The model under review builds one solid part; all positions refer to its coordinate system, in mm. Coordinates: 2 decimals unless noted, no trailing zeros. Loops run counter-clockwise (first coordinate to the right, second up) from the corner with the lowest first, then second, coordinate; pieces in that order, holes last. Notation, with made-up numbers: M 57.5,-14 L 89.5,-14 A27 cw 89.5,8 Z; hole C 4.25,66 d2. An arc over 180 degrees is marked long. Return JSON: item names as keys, results as strings.
```python
from build123d import *

# Parameters (mm, degrees)
F2_DEPTH = 11
F4_DEPTH = 7.1505523714


with BuildPart() as f2:
    # F1 (on Front) → F2 (new body)
    with BuildSketch(Plane.XZ):
        with BuildLine():
            Line((14.506585896, 14), (14.506585896, 20.0424585491))
            Line((14.506585896, 20.0424585491), (-19.4195080549, 20.0424585491))
            Line((-19.4195080549, 20.0424585491), (-19.4195080549, -20.0424585491))
            Line((-19.4195080549, -20.0424585491), (14.506585896, -20.0424585491))
            Line((14.506585896, -20.0424585491), (14.506585896, -14))
            Line((14.506585896, -14), (0, -14))
            ThreePointArc((0, -14), (-14, 0), (0, 14))
            Line((0, 14), (14.506585896, 14))
        make_face()
    extrude(amount=F2_DEPTH)

    # F3 (on face) → F4 (cut, through all)
    with BuildSketch(Plane(origin=(0, 0, -20.0424585491), x_dir=(1, 0, 0), z_dir=(0, 0, -1))):
        with BuildLine():
            Line((-2.4564610794, 8.5), (-2.4564610794, 2.5))
            ThreePointArc((-2.4564610794, 2.5), (-0.3351407359, 3.3786796564), (0.5435389206, 5.5))
            ThreePointArc((0.5435389206, 5.5), (-0.3351407359, 7.6213203436), (-2.4564610794, 8.5))
        make_face()
        with BuildLine():
            ThreePointArc((-2.4564610794, 8.5), (-5.4564610794, 5.5), (-2.4564610794, 2.5))
            Line((-2.4564610794, 2.5), (-2.4564610794, 8.5))
        make_face()
    extrude(amount=-F4_DEPTH, mode=Mode.SUBTRACT)


solid = f2.part
```
1. Add section C-C on y = -5. Give the boundary of the cut face in (x, z), plus the area to 3 significant figures.
Check values:
{"outline": "M -19.42,-20.04 L -5.41,-20.04 L -5.41,-12.91 A14 cw 0,14 L 14.51,14 L 14.51,20.04 L -19.42,20.04 Z; M 0.5,-20.04 L 14.51,-20.04 L 14.51,-14 L 0.5,-14 Z", "area": "608 mm²"}
2. Add section A-A on x = 10. Give the boundary of the cut face in (y, z), plus the area to 3 significant figures.
Check values:
{"outline": "M -11,-20.04 L 0,-20.04 L 0,-14 L -11,-14 Z; M -11,14 L 0,14 L 0,20.04 L -11,20.04 Z", "area": "133 mm²"}
3. To check wall thickness, follow line 1 (Z direction, x = 8, y = -5.25); line 2 (X direction, y = -5.75, z = -18); line 3 (Z direction, x = -13, y = -10). State the ranges of each line that lie inside material, in increasing order.
Check values:
{"line 1": "-20.04 to -14, 14 to 20.04", "line 2": "-19.42 to -5.45, 0.53 to 14.51", "line 3": "-20.04 to -5.2, 5.2 to 20.04"}
4. Insertion check: pin 1 Ø3 at (y, z) = (-9.5, -1) entering from +X (3 decimals); pin 2 Ø1 at (y, z) = (-8.5, 9.5) entering from +X. Each pin has a flat end and moves straight along its axis. Give the tip position at first contact, or say it passes through.
Check values:
{"pin 1": "x = -13.775", "pin 2": "x = -9.8"}
5. Add section B-B on z = -17. Give the boundary of the cut face in (x, y).
Check values:
{"outline": "M -19.42,-11 L 14.51,-11 L 14.51,0 L -19.42,0 Z; hole C -2.46,-5.5 d6"}
6. The part is to be moulded in two halves that separate along Z. For faces 1 (the face through (7, -5, 14)), 2 (the face through (7, -5, -14)), 3 (the face through (-19.42, -5, 0)), 4 (the face through (-3, -9, -20.042)), say which applies: released by +Z, released by -Z, zero draft, split by the parting line, or undercut.
Check values:
{"face 1": "undercut", "face 2": "undercut", "face 3": "zero draft", "face 4": "released by -Z"}
7. Add section D-D on x = -2. Give the boundary of the cut face in (y, z).
Check values:
{"outline": "M -11,-20.04 L -8.47,-20.04 L -8.47,-13.86 L -11,-13.86 Z; M -11,13.86 L 0,13.86 L 0,20.04 L -11,20.04 Z; M -2.53,-20.04 L 0,-20.04 L 0,-13.86 L -2.53,-13.86 Z"}
